Part model, mm, in its own coordinate system. Face numbers are marked on the shaded views. Round coordinates to 2 decimals unless told otherwise and drop trailing zeros. Write each loop counter-clockwise with the first axis right and the second up, starting at its lowest first coordinate (ties: lowest second). Pieces come first, ordered by that corner, then holes. Notation, with made-up numbers: M 10.25,21.5 L 38.25,21.5 A11 ccw 38.25,31.5 Z; hole C 2,76.5 d6. An arc over 180 degrees is marked long. Use one line per item in the form item = value. Start each with the question number.
Item 1: Mould opens along X. For the marked faces 1 and 2 say: +X half, -X half, draft (parallel to the pull), parting line (faces both ways), or undercut.
Item 2: Cut at D-D, the plane z = 0. Give the cut face in (x, y), then the cut area to 3 significant figures.
Item 3: Probe L1, parallel to Y at x = -3, z = -13.5; L2, parallel to Z at x = -33, y = 28; L3, parallel to Z at x = -5, y = -3.9. List the from-to ranges inside material, lowest first.
Item 4: Cut at B-B, the plane z = 40. Give the cut face in (x, y), then the cut area to 3 significant figures.
Item 5: Flat gauge pins, fed straight in: pin 1 Ø2 at (x, y) = (-38, 27) entering from -Z; pin 2 Ø7.5 at (x, z) = (-37.5, 13.5) entering from +Y; pin 3 Ø6 at (x, z) = (-30.5, 6) entering from +Y; pin 4 Ø12 at (x, z) = (-9, -14) entering from -Y. Where does each tip first touch, or does it go through?
Item 6: Cut at C-C, the plane z = -50. Give the cut face in (x, y).
Item 7: Cut at A-A, the plane x = 15. Give the cut face in (y, z), then the cut area to 3 significant figures.
from build123d import *

# Parameters (mm, degrees)
SWEEP_1_PROFILE_R   = 11.5
SWEEP_1_PROFILE_R_2 = 9
EXTRUDE_1_DEPTH     = 5
SKETCH_31_R         = 1.7
CUT_EXTRUDE_1_DEPTH = 26
FILLET_1_R          = 0.5
SKETCH_32_R         = 11.5
SKETCH_32_R_2       = 9
EXTRUDE_2_DEPTH     = 5
EXTRUDE_START       = -2
SKETCH_33_R         = 1.5
EXTRUDE_3_DEPTH     = 2
SKETCH_34_W         = 12
SKETCH_34_H         = 40
CUT_EXTRUDE_2_DEPTH = 2
SKETCH_35_R         = 10.8
SKETCH_35_R_2       = 9
EXTRUDE_4_DEPTH     = 1


with BuildPart() as part:
    # 扫描-薄件1: sweep along a path in 草图1
    with BuildLine(Plane.XY) as sweep_1_path:
        Line((-40, 27.5), (-27.5, 27.5))
        ThreePointArc((-27.5, 27.5), (-8.054563517, 19.445436483), (0, 0))
    # 扫描-薄件1 profile (on start of the path) → 扫描-薄件1 (sweep)
    with BuildSketch(Plane(origin=(-40, 27.5, 0), x_dir=(0, 1, 0), z_dir=(1, 0, 0))):
        Circle(SWEEP_1_PROFILE_R)
        Circle(SWEEP_1_PROFILE_R_2, mode=Mode.SUBTRACT)
    sweep(path=sweep_1_path.line)

    # 草图30 → 凸台-拉伸1 (add, symmetric)
    with BuildSketch(Plane.ZY.offset(40)):
        with BuildLine():
            ThreePointArc((-10.781929326, 23.5), (-11.5, 27.5), (-10.781929326, 31.5))
            Line((-10.781929326, 31.5), (-18, 31.5))
            Line((-18, 31.5), (-18, 23.5))
            Line((-18, 23.5), (-10.781929326, 23.5))
        make_face()
        with BuildLine():
            Line((18, 31.5), (10.781929326, 31.5))
            ThreePointArc((10.781929326, 31.5), (11.319058867, 29.531971056), (11.5, 27.5))
            ThreePointArc((11.5, 27.5), (11.319058867, 25.468028944), (10.781929326, 23.5))
            Line((10.781929326, 23.5), (18, 23.5))
            Line((18, 23.5), (18, 31.5))
        make_face()
    extrude(amount=EXTRUDE_1_DEPTH, both=True)

    # 草图31 → 切除-拉伸1 (cut)
    with BuildSketch(Plane(origin=(0, 31.5, 0), x_dir=(1, 0, 0), z_dir=(0, 1, 0))):
        with Locations(Location((-40, 14, 0), (0, 0, 180))):
            Circle(SKETCH_31_R)
        with Locations(Location((-40, -14, 0), (0, 0, 180))):
            Circle(SKETCH_31_R)
    extrude(amount=-CUT_EXTRUDE_1_DEPTH, mode=Mode.SUBTRACT)

    # 圆角1
    fillet_1_edges = [part.edges().sort_by_distance(p)[0] for p in [
        (-35, 27.5, -18),
        (-40, 31.5, -18),
        (-40, 23.5, -18),
        (-42.5, 23.5, -10.781929326),
        (-45, 27.5, -11.5),
        (-42.5, 31.5, -10.781929326),
        (-45, 27.5, -18),
        (-35, 27.5, -11.5),
        (-42.5, 31.5, 10.781929326),
        (-45, 27.5, 11.5),
        (-42.5, 23.5, 10.781929326),
        (-45, 27.5, 18),
        (-40, 23.5, 18),
        (-40, 31.5, 18),
        (-35, 27.5, 11.5),
        (-35, 27.5, 18),
    ]]
    fillet(fillet_1_edges, radius=FILLET_1_R)

    # 草图32 → 凸台-拉伸2 (add)
    with BuildSketch(Plane.XZ):
        Circle(SKETCH_32_R)
        Circle(SKETCH_32_R_2, mode=Mode.SUBTRACT)
    extrude(amount=EXTRUDE_2_DEPTH)

    # 草图33 → 凸台-拉伸3 (add)
    with BuildSketch(Plane.XZ.offset(5).offset(EXTRUDE_START)):
        with BuildLine():
            Line((-9, -7.158910532), (-9, -53))
            Line((-9, -53), (19, -53))
            Line((19, -53), (19, 53))
            Line((19, 53), (-9, 53))
            Line((-9, 53), (-9, 7.158910532))
            ThreePointArc((-9, 7.158910532), (11.5, 0), (-9, -7.158910532))
        make_face()
        with Locations((-5, 50)):
            Circle(SKETCH_33_R, mode=Mode.SUBTRACT)
        with Locations((15, 50)):
            Circle(SKETCH_33_R, mode=Mode.SUBTRACT)
        with Locations((-5, -50)):
            Circle(SKETCH_33_R, mode=Mode.SUBTRACT)
        with Locations((15, -50)):
            Circle(SKETCH_33_R, mode=Mode.SUBTRACT)
    extrude(amount=EXTRUDE_3_DEPTH)

    # 草图34 → 切除-拉伸2 (cut)
    with BuildSketch(Plane.XZ.offset(5)):
        with Locations((5, 33)):
            Rectangle(SKETCH_34_W, SKETCH_34_H)
        with Locations((5, -33)):
            Rectangle(SKETCH_34_W, SKETCH_34_H)
    extrude(amount=-CUT_EXTRUDE_2_DEPTH, mode=Mode.SUBTRACT)

    # 草图35 → 凸台-拉伸4 (add)
    with BuildSketch(Plane.XZ.offset(5)):
        Circle(SKETCH_35_R)
        Circle(SKETCH_35_R_2, mode=Mode.SUBTRACT)
    extrude(amount=EXTRUDE_4_DEPTH)


solid = part.part
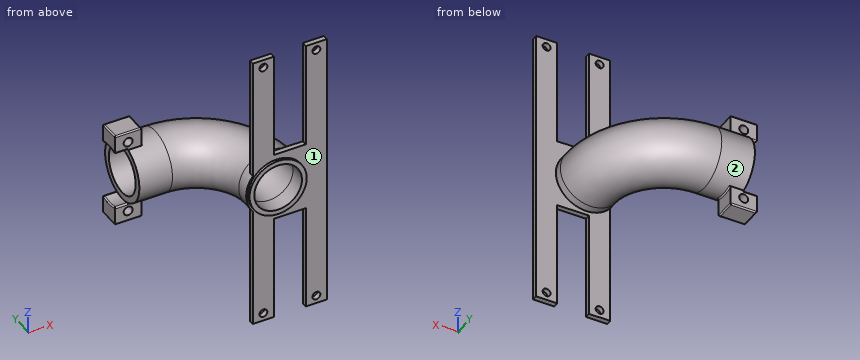
Model answer:
q1.face_1 = draft
q1.face_2 = undercut
q2.outline = M -40,16 L -27.5,16 A16 cw -11.5,0 L -11.5,-5 L -10.8,-5 L -10.8,-6 L -9,-6 L -9,0 A18.5 ccw -27.5,18.5 L -40,18.5 Z; M -40,36.5 L -27.5,36.5 A36.5 cw 9,0 L 9,-6 L 10.8,-6 L 10.8,-5 L 19,-5 L 19,-3 L 11.5,-3 L 11.5,0 A39 ccw -27.5,39 L -40,39 Z
q2.area = 322 mm²
q3.L1 = -5 to -3
q3.L2 = -11.49 to -8.99, 8.99 to 11.49
q3.L3 = -53 to -51.5, -48.5 to -7.48, 7.48 to 48.5, 51.5 to 53
q4.outline = M -9,-5 L -1,-5 L -1,-3 L -9,-3 Z; M 11,-5 L 19,-5 L 19,-3 L 11,-3 Z
q4.area = 32.0 mm²
q5.pin_1 = -18
q5.pin_2 = 33.6
q5.pin_3 = 38.6
q5.pin_4 = -6
q6.outline = M -9,-5 L -6.5,-5 L -6.5,-3 L -9,-3 Z; M -3.5,-5 L -1,-5 L -1,-3 L -3.5,-3 Z; M 11,-5 L 13.5,-5 L 13.5,-3 L 11,-3 Z; M 16.5,-5 L 19,-5 L 19,-3 L 16.5,-3 Z
q7.outline = M -5,-53 L -3,-53 L -3,-51.5 L -5,-51.5 Z; M -5,-48.5 L -3,-48.5 L -3,48.5 L -5,48.5 Z; M -5,51.5 L -3,51.5 L -3,53 L -5,53 Z
q7.area = 200 mm²
